Could you check a few things on this model? Use its own coordinates, in mm. A direction names the side the tool comes from. Coordinates: 2 decimals unless noted, no trailing zeros. Write each loop counter-clockwise with the first axis right and the second up, starting at its lowest first coordinate (ties: lowest second). Pieces come first, ordered by that corner, then holes.
```python
from build123d import *
from build123d.topology import SkipClean

# Parameters (mm, degrees)
CUT_EXTRUDE1_DEPTH = 15
SKETCH3_R          = 3.0000000000000018
CUT_EXTRUDE2_DEPTH = 15
CIRPATTERN2_COUNT  = 6
FILLET1_R          = 1
CHAMFER1_SIZE      = 2
SCALE1_SCALE       = 2


# Some blends are built 0.0001 mm under size
with BuildPart() as part:
    # Sketch1 → Revolve1 (revolve)
    with BuildSketch(Plane.XY, mode=Mode.PRIVATE) as revolve1_sk:
        Polygon((0, 31.5), (0, 34), (3.5, 34), (3.5, 47), (8, 47), (8.000000000000004, 30.499999999999993), (13.000000000000005, 30.499999999999993), (13.000000000000005, 23.499999999999996), (35, 23.49999999999999), (35, 17.000000000000004), (36.00000000000001, 17.000000000000007), (36.00000000000001, 12.500000000000007), (14.000000000000005, 12.5), (14.000000000000005, 14.5), (9.500000000000005, 14.500000000000002), (9.500000000000005, 27.07007724752754), align=None)
    revolve(revolve1_sk.sketch.rotate(Axis((0, 0, 0), (1, 0, 0)), 90), axis=Axis((0, 0, 0), (1, 0, 0)))

    # Sketch2 → Cut-Extrude1 (cut)
    with BuildSketch(Plane(origin=(35, 0, 0), x_dir=(0, 0, -1), z_dir=(1, 0, 0))):
        with BuildLine():
            Line((-7.121328836370207, 22.395014525654634), (-5.151599583757172, 16.200648805792717))
            ThreePointArc((-5.151599583757172, 16.200648805792717), (-6.51e-15, 17), (5.151599583757166, 16.200648805792717))
            Line((5.151599583757166, 16.200648805792717), (7.121328836370199, 22.395014525654634))
            ThreePointArc((7.121328836370199, 22.395014525654634), (-3.78e-15, 23.499999999999996), (-7.121328836370207, 22.395014525654634))
        make_face()
    cut_extrude1 = extrude(amount=-CUT_EXTRUDE1_DEPTH, mode=Mode.SUBTRACT)

    # Sketch3 → Cut-Extrude2 (cut)
    with BuildSketch(Plane(origin=(8.000000000000002, 0, 0), x_dir=(0, 0, -1), z_dir=(1, 0, 0))):
        with Locations((0, 40.5)):
            Circle(SKETCH3_R)
    cut_extrude2 = extrude(amount=-CUT_EXTRUDE2_DEPTH, mode=Mode.SUBTRACT)

    # CirPattern2: Cut-Extrude1, Cut-Extrude2 ×6 about axis
    with SkipClean():  # the faces are left unmerged after this step: merging them gives an invalid solid
        cirpattern2_axis = Axis((0, -8.4e-16, -2.024e-14), (1, 0, 0))
        add([cut_extrude1.rotate(cirpattern2_axis, i * 360 / CIRPATTERN2_COUNT) for i in range(1, CIRPATTERN2_COUNT)], mode=Mode.SUBTRACT)
        add([cut_extrude2.rotate(cirpattern2_axis, i * 360 / CIRPATTERN2_COUNT) for i in range(1, CIRPATTERN2_COUNT)], mode=Mode.SUBTRACT)

    # Fillet1
    fillet1_edges = [part.edges().sort_by_distance(p)[0] for p in [
        (36.00000000000001, -3.97e-15, -17.000000000000007),
        (13.000000000000005, -7.12e-15, -30.499999999999993),
        (8.000000000000004, -7.12e-15, -30.499999999999993),
    ]]
    fillet(fillet1_edges, radius=FILLET1_R - 0.0001)  # a hair under: the kernel refuses the full size

    # Chamfer1
    # the kernel refuses this chamfer: 2 mm, written as the material it takes off along each edge
    with BuildSketch(Plane(origin=(35, -8.761174115451754, -7.988842125078546), x_dir=(0.027495876610585633, -0.6735319368685933, 0.7386465371119375), z_dir=(0, -0.7389259125032596, -0.6737866842192901))) as chamfer1_piece_1_section:
        Polygon((CHAMFER1_SIZE * 0.999621916911, CHAMFER1_SIZE * 0.0274958766106), (-CHAMFER1_SIZE * 0.0274958766106, CHAMFER1_SIZE * 0.999621916911), (0, 0), align=None)
    chamfer1_piece_1 = extrude(amount=16.786731951863647, mode=Mode.PRIVATE)
    chamfer1_piece_1 = chamfer1_piece_1 - Plane(origin=(34.34095626935287, 0, 0), x_dir=(0, 1.1e-16, 1), z_dir=(1, 0, 0)) * Cylinder(17.000000000000004, 42, mode=Mode.PRIVATE)
    add(chamfer1_piece_1, mode=Mode.SUBTRACT)
    with BuildSketch(Plane(origin=(35, -6.131210705649978, -27.979468717509512), x_dir=(-0.9996219169112968, -0.026858575913627898, 0.005885586672240668), z_dir=(0, 0.21405342901395988, 0.9768219538520649))) as chamfer1_piece_2_section:
        Polygon((CHAMFER1_SIZE * 0.999621916911, -CHAMFER1_SIZE * 0.0274958766106), (-CHAMFER1_SIZE * 0.0274958766106, -CHAMFER1_SIZE * 0.999621916911), (0, 0), align=None)
    chamfer1_piece_2 = extrude(amount=16.786731951863644, mode=Mode.PRIVATE)
    chamfer1_piece_2 = chamfer1_piece_2 - Plane(origin=(34.34095626935968, 5.449e-14, 2.889e-14), x_dir=(0, -0.21405342901396118, -0.9768219538520647), z_dir=(1, 0, 0)) * Cylinder(17.00000000000007, 42, mode=Mode.PRIVATE)
    add(chamfer1_piece_2, mode=Mode.SUBTRACT)
    with BuildSketch(Plane(origin=(35, 2.537953169415396, -11.581820413499162), x_dir=(0.02749587661058563, -0.9764526339906394, -0.21397249903237056), z_dir=(0, 0.21405342901395968, -0.976821953852065))) as chamfer1_piece_3_section:
        Polygon((CHAMFER1_SIZE * 0.999621916911, CHAMFER1_SIZE * 0.0274958766106), (-CHAMFER1_SIZE * 0.0274958766106, CHAMFER1_SIZE * 0.999621916911), (0, 0), align=None)
    chamfer1_piece_3 = extrude(amount=16.786731951863636, mode=Mode.PRIVATE)
    chamfer1_piece_3 = chamfer1_piece_3 - Plane(origin=(34.34095626935361, 0, 0), x_dir=(0, 1.1e-16, 1), z_dir=(1, 0, 0)) * Cylinder(17.000000000000004, 42, mode=Mode.PRIVATE)
    add(chamfer1_piece_3, mode=Mode.SUBTRACT)
    with BuildSketch(Plane(origin=(35, 21.165325340930252, -19.299518585802748), x_dir=(-0.9996219169112968, -0.018526355531149796, -0.020317415714554633), z_dir=(0, -0.7389259125032593, 0.6737866842192902))) as chamfer1_piece_4_section:
        Polygon((CHAMFER1_SIZE * 0.999621916911, -CHAMFER1_SIZE * 0.0274958766106), (-CHAMFER1_SIZE * 0.0274958766106, -CHAMFER1_SIZE * 0.999621916911), (0, 0), align=None)
    chamfer1_piece_4 = extrude(amount=16.786731951863647, mode=Mode.PRIVATE)
    chamfer1_piece_4 = chamfer1_piece_4 - Plane(origin=(34.340956269359076, -1.572e-14, 5.224e-14), x_dir=(0, 0.7389259125032586, -0.6737866842192912), z_dir=(1, 0, 0)) * Cylinder(17.00000000000007, 42, mode=Mode.PRIVATE)
    add(chamfer1_piece_4, mode=Mode.SUBTRACT)
    with BuildSketch(Plane(origin=(35, 11.299127284867144, -3.592978288420628), x_dir=(0.027495876610585616, -0.3029206971220457, -0.9526190361443074), z_dir=(0, 0.9529793415172187, -0.30303526963277455))) as chamfer1_piece_5_section:
        Polygon((CHAMFER1_SIZE * 0.999621916911, CHAMFER1_SIZE * 0.0274958766106), (-CHAMFER1_SIZE * 0.0274958766106, CHAMFER1_SIZE * 0.999621916911), (0, 0), align=None)
    chamfer1_piece_5 = extrude(amount=16.78673195186364, mode=Mode.PRIVATE)
    chamfer1_piece_5 = chamfer1_piece_5 - Plane(origin=(34.340956269353335, 0, 0), x_dir=(0, 1.1e-16, 1), z_dir=(1, 0, 0)) * Cylinder(17.000000000000004, 42, mode=Mode.PRIVATE)
    add(chamfer1_piece_5, mode=Mode.SUBTRACT)
    with BuildSketch(Plane(origin=(35, 27.296536046580208, 8.679950131706747), x_dir=(-0.9996219169112968, 0.008332220382478566, -0.026203002386795352), z_dir=(0, -0.9529793415172185, -0.3030352696327747))) as chamfer1_piece_6_section:
        Polygon((CHAMFER1_SIZE * 0.999621916911, -CHAMFER1_SIZE * 0.0274958766106), (-CHAMFER1_SIZE * 0.0274958766106, -CHAMFER1_SIZE * 0.999621916911), (0, 0), align=None)
    chamfer1_piece_6 = extrude(amount=16.78673195186364, mode=Mode.PRIVATE)
    chamfer1_piece_6 = chamfer1_piece_6 - Plane(origin=(34.340956269359246, -7.105e-14, 3.11e-15), x_dir=(0, 0.9529793415172191, 0.3030352696327735), z_dir=(1, 0, 0)) * Cylinder(17.00000000000007, 42, mode=Mode.PRIVATE)
    add(chamfer1_piece_6, mode=Mode.SUBTRACT)
    with BuildSketch(Plane(origin=(35, 8.761174115451746, 7.988842125078507), x_dir=(0.027495876610585623, 0.6735319368685936, -0.738646537111937), z_dir=(0, 0.7389259125032592, 0.6737866842192906))) as chamfer1_piece_7_section:
        Polygon((CHAMFER1_SIZE * 0.999621916911, CHAMFER1_SIZE * 0.0274958766106), (-CHAMFER1_SIZE * 0.0274958766106, CHAMFER1_SIZE * 0.999621916911), (0, 0), align=None)
    chamfer1_piece_7 = extrude(amount=16.786731951863654, mode=Mode.PRIVATE)
    chamfer1_piece_7 = chamfer1_piece_7 - Plane(origin=(34.34095626935326, 0, 0), x_dir=(0, 1.1e-16, 1), z_dir=(1, 0, 0)) * Cylinder(17.000000000000004, 42, mode=Mode.PRIVATE)
    add(chamfer1_piece_7, mode=Mode.SUBTRACT)
    with BuildSketch(Plane(origin=(35, 6.131210705649962, 27.97946871750947), x_dir=(0.027495876610585616, -0.9764526339906394, 0.21397249903237028), z_dir=(0, -0.21405342901395943, -0.976821953852065))) as chamfer1_piece_8_section:
        Polygon((CHAMFER1_SIZE * 0.999621916911, CHAMFER1_SIZE * 0.0274958766106), (-CHAMFER1_SIZE * 0.0274958766106, CHAMFER1_SIZE * 0.999621916911), (0, 0), align=None)
    chamfer1_piece_8 = extrude(amount=16.786731951863636, mode=Mode.PRIVATE)
    chamfer1_piece_8 = chamfer1_piece_8 - Plane(origin=(34.34095626952976, 0, 0), x_dir=(0, 1.1e-16, 1), z_dir=(1, 0, 0)) * Cylinder(17.000000000000004, 42, mode=Mode.PRIVATE)
    add(chamfer1_piece_8, mode=Mode.SUBTRACT)
    with BuildSketch(Plane(origin=(35, -2.537953169415392, 11.581820413499123), x_dir=(0.027495876610585623, 0.9764526339906394, 0.21397249903237017), z_dir=(0, -0.2140534290139593, 0.976821953852065))) as chamfer1_piece_9_section:
        Polygon((CHAMFER1_SIZE * 0.999621916911, CHAMFER1_SIZE * 0.0274958766106), (-CHAMFER1_SIZE * 0.0274958766106, CHAMFER1_SIZE * 0.999621916911), (0, 0), align=None)
    chamfer1_piece_9 = extrude(amount=16.786731951863636, mode=Mode.PRIVATE)
    chamfer1_piece_9 = chamfer1_piece_9 - Plane(origin=(34.34095626935359, 0, 0), x_dir=(0, 1.1e-16, 1), z_dir=(1, 0, 0)) * Cylinder(17.000000000000004, 42, mode=Mode.PRIVATE)
    add(chamfer1_piece_9, mode=Mode.SUBTRACT)
    with BuildSketch(Plane(origin=(35, -21.165325340930245, 19.299518585802712), x_dir=(-0.9996219169112968, 0.018526355531149803, 0.020317415714554626), z_dir=(0, 0.7389259125032591, -0.6737866842192906))) as chamfer1_piece_10_section:
        Polygon((CHAMFER1_SIZE * 0.999621916911, -CHAMFER1_SIZE * 0.0274958766106), (-CHAMFER1_SIZE * 0.0274958766106, -CHAMFER1_SIZE * 0.999621916911), (0, 0), align=None)
    chamfer1_piece_10 = extrude(amount=16.786731951863633, mode=Mode.PRIVATE)
    chamfer1_piece_10 = chamfer1_piece_10 - Plane(origin=(34.34095626935918, 1.405e-14, -9.273e-14), x_dir=(0, -0.7389259125032583, 0.6737866842192916), z_dir=(1, 0, 0)) * Cylinder(17.00000000000007, 42, mode=Mode.PRIVATE)
    add(chamfer1_piece_10, mode=Mode.SUBTRACT)
    with BuildSketch(Plane(origin=(35, -11.299127284867144, 3.5929782884205888), x_dir=(0.027495876610585616, 0.30292069712204583, 0.9526190361443074), z_dir=(0, -0.9529793415172187, 0.30303526963277466))) as chamfer1_piece_11_section:
        Polygon((CHAMFER1_SIZE * 0.999621916911, CHAMFER1_SIZE * 0.0274958766106), (-CHAMFER1_SIZE * 0.0274958766106, CHAMFER1_SIZE * 0.999621916911), (0, 0), align=None)
    chamfer1_piece_11 = extrude(amount=16.78673195186364, mode=Mode.PRIVATE)
    chamfer1_piece_11 = chamfer1_piece_11 - Plane(origin=(34.34095626935327, 0, 0), x_dir=(0, 1.1e-16, 1), z_dir=(1, 0, 0)) * Cylinder(17.000000000000004, 42, mode=Mode.PRIVATE)
    add(chamfer1_piece_11, mode=Mode.SUBTRACT)
    with BuildSketch(Plane(origin=(35, -27.296536046580208, -8.679950131706784), x_dir=(-0.9996219169112968, -0.008332220382478562, 0.026203002386795352), z_dir=(0, 0.9529793415172186, 0.30303526963277466))) as chamfer1_piece_12_section:
        Polygon((CHAMFER1_SIZE * 0.999621916911, -CHAMFER1_SIZE * 0.0274958766106), (-CHAMFER1_SIZE * 0.0274958766106, -CHAMFER1_SIZE * 0.999621916911), (0, 0), align=None)
    chamfer1_piece_12 = extrude(amount=16.786731951863636, mode=Mode.PRIVATE)
    chamfer1_piece_12 = chamfer1_piece_12 - Plane(origin=(34.34095626935956, 6.938e-14, -4.359e-14), x_dir=(0, -0.9529793415172191, -0.3030352696327734), z_dir=(1, 0, 0)) * Cylinder(17.00000000000007, 42, mode=Mode.PRIVATE)
    add(chamfer1_piece_12, mode=Mode.SUBTRACT)


with BuildPart() as part_1:
    # Scale1: scaled about (13.438191471, 0, 0)
    add(part.part.scale(SCALE1_SCALE).moved(Location((-13.438191471, 0, 0))))


solid = part_1.part
```
1. I want a section at C-C on y = 40.5. Give the number of separate pieces and of enclosed holes in the cut face, plus the area to 3 significant figures.
Verdict:
separate pieces: 3
enclosed holes: 0
area: 2,690 mm2
2. On a 3-axis mill with a long thin cutter (end or side, diameter ignored), from which of +Z, -Z, +X, -X, +Y, -Y can I reach the whole of each face in a straight line? I mean faces 1 (the face through (14.562, -24, -8)), 2 (the face through (39.7, 8.7, 39.7)), 3 (the face through (39.744, -38.509, 12.245)), 4 (the face through (39.744, 29.994, -27.35)). Say none if no direction works.
Verdict:
face 1: -X
face 2: +X, +Y
face 3: +X, -Y
face 4: -Z, +X
3. I want a section at B-B on y = -81. Please give me the cut outline in (x, z).
Verdict:
outline: (-6.44, -47.7) - (2.56, -47.7) - (2.56, -6) - (-6.44, -6) - close; (-6.44, 6) - (2.56, 6) - (2.56, 47.7) - (-6.44, 47.7) - close
4. For pin 1 (4 mm diameter, centred on x = 0.5, y = -15.5, fed in from -Z); pin 2 (7 mm diameter, centred on y = 23.5, z = 37.5, fed in from +X); pin 3 (3.5 mm diameter, centred on y = -1.5, z = -42, fed in from +X), each with a flat end and sliding along its axis, tell me the tip position at first contact or that it passes through.
Verdict:
pin 1: stops at z = -93.03
pin 2: stops at x = 26.56
pin 3: stops at x = 56.56
5. I want a section at A-A on x = 39.5. Please give me the cut outline in (y, z).
Verdict:
outline: (-44.79, -14.24) arc R47 ccw to (-34.73, -31.67) - (-25.12, -22.91) arc R34 ccw to (-7.28, -33.21) - (-10.06, -45.91) arc R47 ccw to (10.06, -45.91) - (7.28, -33.21) arc R34 ccw to (25.12, -22.91) - (34.73, -31.67) arc R47 ccw to (44.79, -14.24) - (32.4, -10.3) arc R34 ccw to (32.4, 10.3) - (44.79, 14.24) arc R47 ccw to (34.73, 31.67) - (25.12, 22.91) arc R34 ccw to (7.28, 33.21) - (10.06, 45.91) arc R47 ccw to (-10.06, 45.91) - (-7.28, 33.21) arc R34 ccw to (-25.12, 22.91) - (-34.73, 31.67) arc R47 ccw to (-44.79, 14.24) - (-32.4, 10.3) arc R34 ccw to (-32.4, -10.3) - close; hole circle Ø50 at (0, 0)
6. I want a section at D-D on x = 22. Please give me the cut outline in (y, z).
Verdict:
outline: circle Ø94 at (0, 0); hole circle Ø50 at (0, 0)
7. If we mould it in two halves opening along Y, with no side actions, what happens to faces 5 (the face through (54.53, 37.97, 14.14)), 6 (the face through (56.562, -36, 21)), 7 (the face through (26.562, -20, 34))? For each: pulls with the +Y half, pulls with the -Y half, needs draft (parallel to the pull), parting line crosses it, or undercut.
Verdict:
face 5: pulls with the +Y half
face 6: needs draft
face 7: undercut
8. Please list where these lines run through material, in increasing order: line 1 along Y through (x, z) = (49.5, 0); line 2 along Z through (x, y) = (0, 40); line 3 along Y through (x, z) = (-3, 0).
Verdict:
line 1: y = -34 to -25, 25 to 34
line 2: z = -85.06 to -76.13, -64.17 to -40.23, 40.23 to 64.17, 76.13 to 85.06
line 3: y = -94 to -87, -75 to -58.13, 58.13 to 75, 87 to 94
